Design review of the part built by this model. Coordinates are the model's own, in mm. A direction names the side the tool comes from. Coordinates: 2 decimals unless noted, no trailing zeros. Write each loop counter-clockwise with the first axis right and the second up, starting at its lowest first coordinate (ties: lowest second). Pieces come first, ordered by that corner, then holes.
Q1. To check wall thickness, follow probe 1 along X at (y, z) = (1.95, -140); probe 2 along Z at (x, y) = (147, -169.5); probe 3 along X at (y, z) = (-167, -62). State the ranges of each line that lie inside material, in increasing order.
Q2. Machinability: for faces 4 (the face through (2.535, -40.043, -110.299)), 5 (the face through (99, -94, -5)), 6 (the face through (169.404, -192.465, -90.887)), which of the approach directions +Z, -Z, +X, -X, +Y, -Y give a long, thin tool a straight path to every point of the face, cutting with its end or side? Answer none if there is none.
Q3. The part is to be moulded in two halves that separate along Y. For faces 1 (the face through (99, 5, -101)), 2 (the face through (97.77, 2.54, -57.57)), 3 (the face through (195, -94, -101)), say which applies: +Y half, -Y half, draft (parallel to the pull), parting line (faces both ways), or undercut.
Q4. Add section A-A, the plane x = 100. Give the boundary of the cut face in (y, z).
Q5. Add section D-D, the plane z = -60. Give the boundary of the cut face in (x, y), plus the area to 3 significant figures.
Q6. Add section C-C, the plane z = -14.5. Give the boundary of the cut face in (x, y), plus the area to 3 significant figures.
Q7. Add section B-B, the plane y = -23.5. Give the boundary of the cut face in (x, z), plus the area to 3 significant figures.
from build123d import *

# Parameters (mm, degrees)
SKETCH_1_W          = 200
SKETCH_1_H          = 200
EXTRUDE_1_DEPTH     = 5
SKETCH_3_W          = 200
SKETCH_3_H          = 200
SKETCH_3_W_2        = 190
SKETCH_3_H_2        = 190
EXTRUDE_2_DEPTH     = 190
SKETCH_4_W          = 200
SKETCH_4_H          = 200
SKETCH_4_R          = 70
EXTRUDE_3_DEPTH     = 5
SKETCH_5_R          = 3.3
CUT_EXTRUDE_1_DEPTH = 5
SKETCH_7_R          = 5
CUT_EXTRUDE_2_DEPTH = 344.547667726


with BuildPart() as part:
    # 草图1 → 凸台-拉伸1 (new body)
    with BuildSketch(Plane(origin=(0, 0, 0), x_dir=(1, 0, 0), z_dir=(0, 1, 0))):
        with Locations((100, 100)):
            Rectangle(SKETCH_1_W, SKETCH_1_H)
    extrude(amount=EXTRUDE_1_DEPTH)

    # 草图3 → 凸台-拉伸2 (add)
    with BuildSketch(Plane.XZ):
        with Locations((100, -100)):
            Rectangle(SKETCH_3_W, SKETCH_3_H)
        with Locations((100, -100)):
            Rectangle(SKETCH_3_W_2, SKETCH_3_H_2, mode=Mode.SUBTRACT)
    extrude(amount=EXTRUDE_2_DEPTH)

    # 草图4 → 凸台-拉伸3 (add)
    with BuildSketch(Plane.XZ.offset(190)):
        with Locations((100, -100)):
            Rectangle(SKETCH_4_W, SKETCH_4_H)
        with Locations(Location((100, -100, 0), (0, 0, 270))):
            Circle(SKETCH_4_R, mode=Mode.SUBTRACT)
    extrude(amount=EXTRUDE_3_DEPTH)

    # 草图5 → 切除-拉伸1 (cut)
    with BuildSketch(Plane(origin=(0, 5, 0), x_dir=(1, 0, 0), z_dir=(0, 1, 0))):
        with Locations(Location((100, 140, 0), (0, 0, 270))):
            Circle(SKETCH_5_R)
        with Locations(Location((100, 60, 0), (0, 0, 90))):
            Circle(SKETCH_5_R)
    extrude(amount=-CUT_EXTRUDE_1_DEPTH, mode=Mode.SUBTRACT)

    # 草图7 → 切除-拉伸2 (cut, through all)
    with BuildSketch(Plane(origin=(200, 0, 0), x_dir=(0, 0, -1), z_dir=(1, 0, 0))):
        with Locations((110.95, -45)):
            Circle(SKETCH_7_R)
    extrude(amount=-CUT_EXTRUDE_2_DEPTH, mode=Mode.SUBTRACT)


solid = part.part
Here are the results:
1. probe 1: x = 0 to 96.7, 103.3 to 200
1. probe 2: z = -200 to -195, -5 to 0
1. probe 3: x = 0 to 5, 195 to 200
2. face 4: +X, -X
2. face 5: none
2. face 6: -Y
3. face 1: +Y half
3. face 2: draft
3. face 3: undercut
4. outline: (-195, -200) - (5, -200) - (5, -143.3) - (0, -143.3) - (0, -195) - (-190, -195) - (-190, -170) - (-195, -170) - close; (-195, -30) - (-190, -30) - (-190, -5) - (0, -5) - (0, -56.7) - (5, -56.7) - (5, 0) - (-195, 0) - close; (0, -136.7) - (5, -136.7) - (5, -63.3) - (0, -63.3) - close
5. outline: (0, -195) - (42.55, -195) - (42.55, -190) - (5, -190) - (5, 0) - (96.7, 0) - (96.7, 5) - (0, 5) - close; (103.3, 0) - (195, 0) - (195, -190) - (157.45, -190) - (157.45, -195) - (200, -195) - (200, 5) - (103.3, 5) - close
5. area: 3,290 mm2
6. outline: (0, -195) - (200, -195) - (200, 5) - (0, 5) - close; hole (5, -190) - (195, -190) - (195, 0) - (5, 0) - close
6. area: 3,900 mm2
7. outline: (0, -200) - (200, -200) - (200, 0) - (0, 0) - close; hole (5, -195) - (195, -195) - (195, -5) - (5, -5) - close
7. area: 3,900 mm2
